Could you check a few things on this model? Use its own coordinates, in mm. A direction names the side the tool comes from. Coordinates: 2 decimals unless noted, no trailing zeros. Order: outer loops, then holes, each group sorted by start corner. A loop starts at its lowest first (then second) coordinate and runs counter-clockwise, first axis right, second up. Notation, with made-up numbers: (-10.75, -17) -> (41.25, -17) arc R6 cw to (41.25, -8) -> close; hole circle Ø8 at (88.25, -1). An arc over 180 degrees is marked (long way). Use a Markdown table: item, result. Add a question column.
1) Will these pins go through, and if not, where does the flat tip stop? pin 1 Ø0.8 at (x, y) = (47, 29) entering from +Z; pin 2 Ø1.9 at (y, z) = (2.5, -27.5) entering from -X; pin 3 Ø9.5 at (y, z) = (11, -10.5) entering from -X.
2) If we section it at A-A (y = 20.5): Write out the boundary of the cut face in (x, z), plus the area to 3 significant figures.
3) If we section it at C-C (x = 46.99): Write out the boundary of the cut face in (y, z).
4) If I drill on L1, parallel to Y at x = 46.99, z = -2.5; L2, parallel to X at y = 22, z = -8.5; L3, parallel to Z at x = 44.5, y = 4.5, over which ranges is the centre line in solid material (lowest first)? Write a range as [from, to].
5) Which directions (+Z, -Z, +X, -X, +Y, -Y) give clear straight access to the entire face, cutting with the end or side of a thin tool? Please do faces 1 (the flat face through (-50.231, 2.223, -18.783)), 2 (the cylindrical face through (-43.6, 0.22, -10.95)), 3 (the cylindrical face through (-44.87, -0.07, -20.11)).
6) If we section it at D-D (x = -31.5): Write out the boundary of the cut face in (y, z).
7) If we section it at B-B (z = -29.5): Write out the boundary of the cut face in (x, y), plus the area to 3 significant figures.
8) Thinking about a two-plate mould opening in Y: for faces 4 (the flat face through (1, -0.545, -19)), 5 (the cylindrical face through (-47.96, 29.47, -3.76)), 6 (the flat face through (-51.118, 0, -19)), which applies, +Y half, -Y half, draft (parallel to the pull), parting line (faces both ways), or undercut?
```python
from build123d import *

# Parameters (mm, degrees)
BOSS_EXTRUDE1_DEPTH      = 101.6
SKETCH3_W                = 19.05
SKETCH3_H                = 15.24
BOSS_EXTRUDE3_DEPTH      = 2.54
BOSS_EXTRUDE4_DEPTH      = 3.175
SKETCH5_R                = 3.96875
CUT_EXTRUDE1_DEPTH       = 113.522583006
SKETCH18_W               = 3.847197439
SKETCH18_H               = 19.05
BOSS_EXTRUDE9_DEPTH      = 3.630394878
BOSS_EXTRUDE17_DEPTH     = 19.05
SKETCH20_R               = 1.3208
CUT_EXTRUDE7_DEPTH       = 7.62
FILLET3_R                = 2.54
FILLET4_R                = 2.54
CUT_EXTRUDE19_DEPTH      = 119.165702994
FILLET12_R               = 0.508
FILLET24_R               = 1.27
CUT_EXTRUDE20_DEPTH      = 119.230869843
CUT_EXTRUDE20_DEPTH_BACK = 119.230869843
SKETCH41_W               = 159.957489038
SKETCH41_H               = 86.494386596


with BuildPart() as part:
    # Sketch1 → Boss-Extrude1 (new body)
    with BuildSketch(Plane.XY):
        Polygon((-49.440197439, 3.085197439), (-51.308, 1.217394878), (-51.308, -1.217394878), (-49.440197439, -3.085197439), (49.440197439, -3.085197439), (51.308, -1.217394878), (51.308, 1.217394878), (49.440197439, 3.085197439), (48.170197439, 3.085197439), (48.170197439, -0.545197439), (-48.170197439, -0.545197439), (-48.170197439, 3.085197439), align=None)
    extrude(amount=-BOSS_EXTRUDE1_DEPTH)

    # Sketch3 → Boss-Extrude3 (add)
    with BuildSketch(Plane(origin=(0, 0, -101.6), x_dir=(-1, 0, 0), z_dir=(0, 0, -1))):
        with Locations((38.645197439, 7.074802561)):
            Rectangle(SKETCH3_W, SKETCH3_H)
    extrude(amount=-BOSS_EXTRUDE3_DEPTH)

    # Sketch4 → Boss-Extrude4 (add)
    with BuildSketch(Plane(origin=(-29.120197439, 0, 0), x_dir=(0, 0, -1), z_dir=(1, 0, 0))):
        Polygon((99.06, 14.694802561), (83.82, -0.545197439), (99.06, -0.545197439), align=None)
    boss_extrude4 = extrude(amount=-BOSS_EXTRUDE4_DEPTH)

    # Mirror1: Boss-Extrude4 across plane
    add(boss_extrude4.mirror(Plane(origin=(-38.645197439, 0, 0), x_dir=(0, 0, 1), z_dir=(1, 0, 0))))

    # Sketch5 → Cut-Extrude1 (cut, through all)
    with BuildSketch(Plane.XY.offset(-99.06)):
        with Locations((-38.6334, 6.985)):
            Circle(SKETCH5_R)
    extrude(amount=-CUT_EXTRUDE1_DEPTH, mode=Mode.SUBTRACT)

    # Sketch18 → Boss-Extrude9 (add)
    with BuildSketch(Plane(origin=(0, 3.085197439, 0), x_dir=(1, 0, 0), z_dir=(0, 1, 0))):
        with Locations((46.246598719, 9.525)):
            Rectangle(SKETCH18_W, SKETCH18_H)
        with Locations((-46.246598719, 9.525)):
            Rectangle(SKETCH18_W, SKETCH18_H)
    extrude(amount=-BOSS_EXTRUDE9_DEPTH)

    # Sketch39 → Boss-Extrude17 (add)
    with BuildSketch(Plane.XY):
        with BuildLine():
            Line((49.186197439, 3.085197439), (44.323, 3.085197439))
            Line((44.323, 3.085197439), (44.323, 25.325923901))
            Line((44.323, 25.325923901), (43.86013816, 28.041530355))
            ThreePointArc((43.86013816, 28.041530355), (47.275748779, 31.737115215), (49.973524071, 27.489086045))
            Line((49.973524071, 27.489086045), (49.186197439, 25.325923901))
            Line((49.186197439, 25.325923901), (49.186197439, 3.085197439))
        make_face()
    boss_extrude17 = extrude(amount=-BOSS_EXTRUDE17_DEPTH)

    # Mirror5: Boss-Extrude17 across plane
    add(boss_extrude17.mirror(Plane(origin=(0, 0, 0), x_dir=(0, 0, 1), z_dir=(1, 0, 0))))

    # Sketch20 → Cut-Extrude7 (cut)
    with BuildSketch(Plane.XY):
        with Locations((46.99, 0)):
            Circle(SKETCH20_R)
        with Locations((-46.99, 0)):
            Circle(SKETCH20_R)
        with Locations((-46.99, 28.575)):
            Circle(SKETCH20_R)
        with Locations((46.99, 28.575)):
            Circle(SKETCH20_R)
    extrude(amount=-CUT_EXTRUDE7_DEPTH, mode=Mode.SUBTRACT)

    # Fillet3
    fillet3_edges = [part.edges().sort_by_distance(p)[0] for p in [
        (44.323, 25.325923901, -9.525),
        (49.186197439, 25.325923901, -9.525),
        (-49.186197439, 25.325923901, -9.525),
        (-44.323, 25.325923901, -9.525),
    ]]
    fillet(fillet3_edges, radius=FILLET3_R)

    # Fillet4
    fillet4_edges = [part.edges().sort_by_distance(p)[0] for p in [
        (48.678197439, 3.085197439, -19.05),
        (-48.678197439, 3.085197439, -19.05),
        (44.323, -0.545197439, -9.525),
        (46.246598719, -0.545197439, -19.05),
        (-46.246598719, -0.545197439, -19.05),
        (-44.323, -0.545197439, -9.525),
    ]]
    fillet(fillet4_edges, radius=FILLET4_R)

    # Sketch40 → Cut-Extrude19 (cut, through all)
    with BuildSketch(Plane.XY):
        Polygon((-49.36835539, 3.085197439), (-51.1175, 1.336052829), (-51.1175, -1.336052829), (-49.36835539, -3.085197439), (-52.3875, -3.085197439), (-52.3875, 3.085197439), align=None)
        Polygon((52.3875, 3.085197439), (52.3875, -3.085197439), (49.36835539, -3.085197439), (51.1175, -1.336052829), (51.1175, 1.336052829), (49.36835539, 3.085197439), align=None)
    extrude(amount=-CUT_EXTRUDE19_DEPTH, mode=Mode.SUBTRACT)

    # Fillet12
    # the kernel refuses this fillet: 0.508 mm, written as the material it adds along each edge
    with BuildSketch(Plane(origin=(-48.170197439, 3.085197439, -86.180394878), x_dir=(-1, 0, 0), z_dir=(0, 0, -1))) as fillet12_piece_1_section:
        with BuildLine():
            CenterArc((FILLET12_R, FILLET12_R), FILLET12_R, 180, 90)
            Line((0, FILLET12_R), (0, 0))
            Line((0, 0), (FILLET12_R, 0))
        make_face()
    fillet12_piece_1 = extrude(amount=15.419605122, mode=Mode.PRIVATE)
    fillet12_piece_1 = split(fillet12_piece_1, bisect_by=Plane(origin=(-48.284048629, 6.707217092, -91.072414531), z_dir=(0, -0.7071067811865475, -0.7071067811865476)), keep=Keep.TOP, mode=Mode.PRIVATE)
    add(fillet12_piece_1)

    # Fillet24
    fillet24_edges = [part.edges().sort_by_distance(p)[0] for p in [
        (-48.170197439, 3.81, -19.05),
        (-48.170197439, 0.198751337, -19.793948776),
        (-48.170197439, -0.545197439, -52.705),
    ]]
    fillet(fillet24_edges, radius=FILLET24_R)

    # Sketch41 → Cut-Extrude20 (cut, two sides: drawn at the far end of the back side and taken through both)
    with BuildSketch(Plane(origin=(0, -0.545197439, 0), x_dir=(1, 0, 0), z_dir=(0, 1, 0)).offset(-CUT_EXTRUDE20_DEPTH_BACK)):
        with Locations((1.60361347, 81.347193298)):
            Rectangle(SKETCH41_W, SKETCH41_H)
    extrude(amount=CUT_EXTRUDE20_DEPTH + CUT_EXTRUDE20_DEPTH_BACK, mode=Mode.SUBTRACT)


solid = part.part
```
Answer sheet:
| question | item | result |
|---|---|---|
| 1 | pin 1 | z = -7.62 |
| 1 | pin 2 | x = -50.9 |
| 1 | pin 3 | x = -49.19 |
| 2 | outline | (-49.19, -19.05) -> (-44.32, -19.05) -> (-44.32, 0) -> (-49.19, 0) -> close; (44.32, -19.05) -> (49.19, -19.05) -> (49.19, 0) -> (44.32, 0) -> close |
| 2 | area | 185 mm2 |
| 3 | outline | (-3.09, -38.1) -> (-0.55, -38.1) -> (-0.55, -21.59) arc R2.54 cw to (1.99, -19.05) -> (31.75, -19.05) -> (31.75, 0) -> (29.9, 0) -> (29.9, -7.62) -> (27.25, -7.62) -> (27.25, 0) -> (1.32, 0) -> (1.32, -7.62) -> (-1.32, -7.62) -> (-1.32, 0) -> (-3.09, 0) -> close |
| 4 | L1 | [-3.09, -1.32], [1.32, 27.25], [29.9, 31.75] |
| 4 | L2 | [-49.19, -44.32], [44.32, 49.19] |
| 4 | L3 | [-19.05, 0] |
| 5 | face 1 | +Z, -Z, -X |
| 5 | face 2 | +Z, -Z |
| 5 | face 3 | -Z, +Y |
| 6 | outline | (-3.09, -38.1) -> (-0.55, -38.1) -> (-0.55, 0) -> (-3.09, 0) -> close |
| 7 | outline | (-51.12, -1.34) -> (-49.37, -3.09) -> (49.37, -3.09) -> (51.12, -1.34) -> (51.12, 1.34) -> (49.37, 3.09) -> (48.17, 3.09) -> (48.17, -0.55) -> (-46.9, -0.55) arc R1.27 cw to (-48.17, 0.72) -> (-48.17, 3.09) -> (-49.37, 3.09) -> (-51.12, 1.34) -> close |
| 7 | area | 275 mm2 |
| 8 | face 4 | +Y half |
| 8 | face 5 | undercut |
| 8 | face 6 | draft |
